Check sheet for the modelled part. Datum: model origin and axes. Units: mm. A direction names the side the tool comes from. Give positions to 0.01 mm unless a question says otherwise; leave off trailing zeros. Write each loop counter-clockwise with the first axis right and the second up, starting at its lowest first coordinate (ties: lowest second). Pieces come first, ordered by that corner, then holes. Notation, with made-up numbers: (69.25, 12.5) -> (84.25, 12.5) arc R26 cw to (84.25, 30.5) -> close; hole circle Ø6 at (80, -24.5). An arc over 180 degrees is marked (long way). Use a Markdown table: item, result. Add a question column.
1. Set-up check for faces 1 (the flat face through (-20, 0, 8)), 2 (the flat face through (-18, -22.5, 33)), 3 (the flat face through (-5, -12.5, 33)): record each of +Z, -Z, +X, -X, +Y, -Y from which the full face is reachable in a straight line by a thin tool's end or side.
2. Scan lines: probe 1 along Y at (x, z) = (-2, 36); probe 2 along X at (y, z) = (-4.5, 24); probe 3 along Z at (x, y) = (-24, 0). Record each from-to range of solid material in increasing order. Write a range as [from, to].
3. Release check for a two-part mould opening along Y. For faces 4 (the cylindrical face through (-27.745, 0.521, 34.966)), 5 (the flat face through (-35, 0, 55)), 6 (the flat face through (-18, 22.5, 33)) record: released by +Y, released by -Y, zero draft, split by the parting line, or undercut.
4. Cross-section at D-D (y = 17). Enter the section's corners in (x, z).
5. Cross-section at A-A (z = 31). Enter the section's corners in (x, y).
6. Cross-section at B-B (y = 0). Enter the section's corners in (x, z).
7. Gauge pin test, flat ends, axial feed: P1, Ø20, axis at x = -27.5, y = 11, coming from the -Z side; P2, Ø4, axis at x = -29.5, y = 5, coming from the -Z side; P3, Ø7.5, axis at y = -9, z = 9, coming from the -X side; P4, Ø10.5, axis at y = 0, z = 31, coming from the +X side. Record the tip position at first contact, or that the pin passes through.
8. Cross-section at C-C (x = -13). Enter the section's corners in (y, z).
from build123d import *

# Parameters (mm, degrees)
F1_DEPTH = 22.5
F2_SIZE  = 20
F3_W     = 10
F3_H     = 25
F4_DEPTH = 65.001
F5_R     = 4
F6_DEPTH = 45.001


with BuildPart() as f1:
    # F0 (on Front) → F1 (new body, symmetric)
    with BuildSketch(Plane.XZ):
        Polygon((-20, 0), (0, 0), (0, 65), (-45, 65), (-45, 15), (-20, 15), align=None)
    extrude(amount=F1_DEPTH, both=True)

    # F2
    f2_edges = [f1.edges().sort_by_distance(p)[0] for p in [
        (-45, 0, 65),
    ]]
    chamfer(f2_edges, length=F2_SIZE)

    # F3 (on face) → F4 (cut, through all)
    with BuildSketch(Plane.XY.offset(65)):
        with Locations((-5, 0)):
            Rectangle(F3_W, F3_H)
    extrude(amount=-F4_DEPTH, mode=Mode.SUBTRACT)

    # F5 (on face) → F6 (cut, through all)
    with BuildSketch(Plane(origin=(-45, 0, 0), x_dir=(0, -1, 0), z_dir=(-1, 0, 0))):
        with Locations((0, 31)):
            Circle(F5_R)
    extrude(amount=-F6_DEPTH, mode=Mode.SUBTRACT)


solid = f1.part
Worked answers:
| question | item | result |
|---|---|---|
| 1 | face 1 | -Z, -X, +Y, -Y |
| 1 | face 2 | +Z, -Z, +X, -X, -Y |
| 1 | face 3 | +Z, -Z, +X |
| 2 | probe 1 | y = [-22.5, -12.5], [12.5, 22.5] |
| 2 | probe 2 | x = [-45, -10] |
| 2 | probe 3 | z = [15, 27], [35, 65] |
| 3 | face 4 | undercut |
| 3 | face 5 | zero draft |
| 3 | face 6 | released by +Y |
| 4 | outline | (-45, 15) -> (-20, 15) -> (-20, 0) -> (0, 0) -> (0, 65) -> (-25, 65) -> (-45, 45) -> close |
| 5 | outline | (-45, -22.5) -> (0, -22.5) -> (0, -12.5) -> (-10, -12.5) -> (-10, -4) -> (-45, -4) -> close; (-45, 4) -> (-10, 4) -> (-10, 12.5) -> (0, 12.5) -> (0, 22.5) -> (-45, 22.5) -> close |
| 6 | outline | (-45, 15) -> (-20, 15) -> (-20, 0) -> (-10, 0) -> (-10, 27) -> (-45, 27) -> close; (-45, 35) -> (-10, 35) -> (-10, 65) -> (-25, 65) -> (-45, 45) -> close |
| 7 | P1 | stops at z = 0 |
| 7 | P2 | stops at z = 15 |
| 7 | P3 | stops at x = -20 |
| 7 | P4 | stops at x = -10 |
| 8 | outline | (-22.5, 0) -> (22.5, 0) -> (22.5, 65) -> (-22.5, 65) -> close; hole circle Ø8 at (0, 31) |
